Here's how the part is built. I have some questions about the finished solid (model axes, mm). Face numbers are marked on the shaded views. A direction names the side the tool comes from. Round coordinates to 2 decimals unless told otherwise and drop trailing zeros. Write each loop counter-clockwise with the first axis right and the second up, starting at its lowest first coordinate (ties: lowest second). Pieces come first, ordered by that corner, then holes. Notation, with made-up numbers: (29, -25) - (72, -25) arc R20 cw to (72, 14) - close; hole circle Ø8 at (50.5, 56.5). An arc over 180 degrees is marked (long way). One line per item, written item: value. Start each with the question number.
Item 1: If I drill on line 1 (Z direction, x = 6.5, y = 0); line 2 (Z direction, x = 0, y = 5); line 3 (Z direction, x = -3.25, y = -6), over which ranges is the centre line in solid material (lowest first)?
Item 2: For P1, Ø1, axis at x = 0, z = 5.5, coming from the +Y side; P2, Ø8, axis at x = 6, z = 13, coming from the -Y side; P3, Ø3, axis at x = 0.5, z = 3.5, coming from the -Y side, each with a flat end and sliding along its axis, tell me the tip position at first contact or that it passes through.
Item 3: Imagine slicing it at D-D, the plane y = 6.75. Please give me the cut outline in (x, z), then the cut area to 3 significant figures.
Item 4: Imagine slicing it at B-B, the plane z = 12.25. Please give me the cut outline in (x, y), then the cut area to 3 significant figures.
Item 5: For the marked faces 4, 5, 6 and 7, which set-ups out of +Z, -Z, +X, -X, +Y, -Y let a thin tool reach every point of the face, with its end or its side?
Item 6: Imagine slicing it at A-A, the plane y = 0. Please give me the cut outline in (x, z), then the cut area to 4 significant figures.
Item 7: Thinking about a two-plate mould opening in X: for the marked faces 1, 2 and 3, which applies, released by +X, released by -X, zero draft, split by the parting line, or undercut?
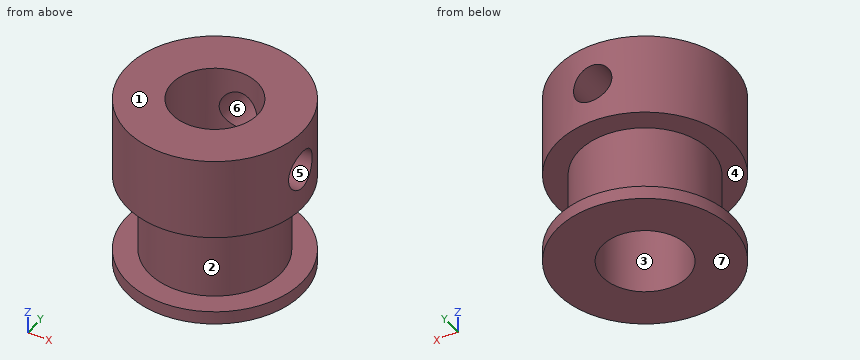
```python
from build123d import *

# Parameters (mm, degrees)
SKETCH2_R               = 8
SKETCH2_R_2             = 3.9
BOSS_EXTRUDE1_DEPTH     = 16
SKETCH3_OUTSIDE_W       = 23.542
SKETCH3_OUTSIDE_H       = 23.542
SKETCH3_OUTSIDE_R       = 6
CUT_EXTRUDE1_DEPTH      = 7.3
CUT_EXTRUDE2_REACH      = 26
CUT_EXTRUDE2_END_RADIUS = 3.9
SKETCH6_R               = 1.75
CUT_EXTRUDE3_REACH      = 26
CUT_EXTRUDE3_END_RADIUS = 3.9
SKETCH5_R               = 1.75


with BuildPart() as part:
    # Sketch2 → Boss-Extrude1 (new body)
    with BuildSketch(Plane.XY):
        Circle(SKETCH2_R)
        Circle(SKETCH2_R_2, mode=Mode.SUBTRACT)
    extrude(amount=BOSS_EXTRUDE1_DEPTH)

    # Sketch3 outside → Cut-Extrude1 (cut)
    with BuildSketch(Plane.XY.offset(1.2)):
        Rectangle(SKETCH3_OUTSIDE_W, SKETCH3_OUTSIDE_H)
        with Locations(Location((0, 0, 0), (0, 0, 180))):
            Circle(SKETCH3_OUTSIDE_R, mode=Mode.SUBTRACT)
    extrude(amount=CUT_EXTRUDE1_DEPTH, mode=Mode.SUBTRACT)

    # Cut-Extrude2: up to this cylinder (the profile starts outside it)
    cut_extrude2_end = Plane(origin=(0, 0, 12.25), z_dir=(0, 0, -1)) * Cylinder(CUT_EXTRUDE2_END_RADIUS, 60.8, mode=Mode.PRIVATE)
    # Sketch6 → Cut-Extrude2 (cut, up to the surface)
    with BuildSketch(Plane(origin=(8, 0, 0), x_dir=(0, 0, -1), z_dir=(1, 0, 0)), mode=Mode.PRIVATE) as cut_extrude2_sk1:
        with Locations((-12.25, 0)):
            Circle(SKETCH6_R)
    cut_extrude2_tool1 = extrude(cut_extrude2_sk1.sketch, amount=-CUT_EXTRUDE2_REACH, mode=Mode.PRIVATE) - cut_extrude2_end
    add(cut_extrude2_tool1.solids().sort_by_distance((8, 0, 12.25))[0], mode=Mode.SUBTRACT)

    # Cut-Extrude3: up to this cylinder (the profile starts outside it)
    cut_extrude3_end = Plane(origin=(0, 0, 12.25), z_dir=(0, 0, -1)) * Cylinder(CUT_EXTRUDE3_END_RADIUS, 60.8, mode=Mode.PRIVATE)
    # Sketch5 → Cut-Extrude3 (cut, up to the surface)
    with BuildSketch(Plane(origin=(0, 8, 0), x_dir=(1, 0, 0), z_dir=(0, 1, 0)), mode=Mode.PRIVATE) as cut_extrude3_sk1:
        with Locations(Location((0, -12.25, 0), (0, 0, 270))):
            Circle(SKETCH5_R)
    cut_extrude3_tool1 = extrude(cut_extrude3_sk1.sketch, amount=-CUT_EXTRUDE3_REACH, mode=Mode.PRIVATE) - cut_extrude3_end
    add(cut_extrude3_tool1.solids().sort_by_distance((0, 8, 12.25))[0], mode=Mode.SUBTRACT)


solid = part.part
```
Values follow:
1. line 1: z = 0 to 1.2, 8.5 to 10.5, 14 to 16
1. line 2: z = 0 to 10.5, 14 to 16
1. line 3: z = 0 to 1.2, 8.5 to 16
2. P1: stops at y = 6
2. P2: stops at y = -7.75
2. P3: stops at y = -6
3. outline: (-4.29, 0) - (4.29, 0) - (4.29, 1.2) - (-4.29, 1.2) - close; (-4.29, 8.5) - (4.29, 8.5) - (4.29, 16) - (-4.29, 16) - close; hole circle Ø3.5 at (0, 12.25)
3. area: 65.1 mm^2
4. outline: (-1.75, 3.49) - (-1.75, 7.81) arc R8 ccw (long way) to (7.81, -1.75) - (3.49, -1.75) arc R3.9 cw (long way) to start; (1.75, 3.49) arc R3.9 cw to (3.49, 1.75) - (7.81, 1.75) arc R8 ccw to (1.75, 7.81) - close
4. area: 124 mm^2
5. face 4: none
5. face 5: +X
5. face 6: +Y
5. face 7: -Z, +X, -X, +Y, -Y
6. outline: (-8, 0) - (-3.9, 0) - (-3.9, 16) - (-8, 16) - (-8, 8.5) - (-6, 8.5) - (-6, 1.2) - (-8, 1.2) - close; (3.9, 0) - (8, 0) - (8, 1.2) - (6, 1.2) - (6, 8.5) - (8, 8.5) - (8, 10.5) - (3.9, 10.5) - close; (3.9, 14) - (8, 14) - (8, 16) - (3.9, 16) - close
6. area: 87.65 mm^2
7. face 1: zero draft
7. face 2: split by the parting line
7. face 3: undercut
